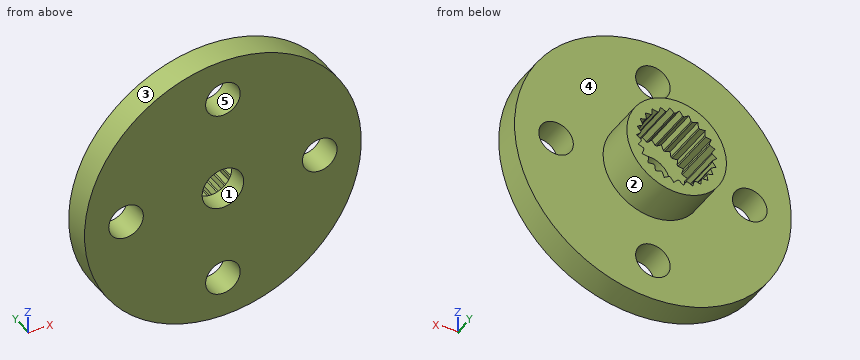
```python
from build123d import *

# Parameters (mm, degrees)
M3_TAPPED_HOLE1_D  = 2.5
CUT_EXTRUDE1_DEPTH = 3.5


with BuildPart() as part:
    # Sketch1 → Revolve1 (revolve)
    with BuildSketch(Plane.XY, mode=Mode.PRIVATE) as revolve1_sk:
        Polygon((2.345142076, 2), (1.5, 2), (1.5, 0), (10, 0), (10, 2), (3.6, 2), (3.6, 5), (2.345142076, 5), align=None)
    revolve(revolve1_sk.sketch.rotate(Axis((0, 6.795271061, 0), (0, -1, 0)), 90), axis=Axis((0, 6.795271061, 0), (0, -1, 0)))

    # M3 Tapped Hole1 (through all)
    with Locations(Plane(origin=(0, 2, 0), x_dir=(1, 0, 0), z_dir=(0, 1, 0))):
        with Locations((-7, 0), (0, 7), (7, 0), (0, -7)):
            Hole(M3_TAPPED_HOLE1_D / 2)

    # Sketch5 → Cut-Extrude1 (cut)
    with BuildSketch(Plane(origin=(0, 5, 0), x_dir=(1, 0, 0), z_dir=(0, 1, 0))):
        Polygon((-1.365561553, 2.212519298), (-1.76486465, 2.301141622), (-1.782802347, 1.892515731), (-1.855371341, 1.821427239), (-2.264280127, 1.811914873), (-2.18390601, 1.410870135), (-2.237353692, 1.324480448), (-2.632103873, 1.217386217), (-2.458088994, 0.847229896), (-2.489309178, 0.750559669), (-2.846959309, 0.552107499), (-2.589416781, 0.234351734), (-2.596595063, 0.133019089), (-2.896359819, -0.1452577), (-2.570257076, -0.392146098), (-2.552976281, -0.492252076), (-2.777434424, -0.834181049), (-2.401723373, -0.995853825), (-2.360987798, -1.08891534), (-2.497094635, -1.474624828), (-2.093610237, -1.541686147), (-2.031787285, -1.622294803), (-2.071632783, -2.029368772), (-1.663824084, -1.997921274), (-1.584506681, -2.061392388), (-1.525775164, -2.466173179), (-1.137342523, -2.338044479), (-1.045140308, -2.380689341), (-0.891245038, -2.759652566), (-0.544762749, -2.542289037), (-0.445034179, -2.561629282), (-0.20491899, -2.892750976), (0.079476656, -2.598784997), (0.180935719, -2.593696641), (0.493316205, -2.857733214), (0.699097167, -2.504249019), (0.79639029, -2.475027779), (1.162881655, -2.656634385), (1.278088691, -2.264175191), (1.365561553, -2.212519298), (1.76486465, -2.301141622), (1.782802347, -1.892515731), (1.855371341, -1.821427239), (2.264280127, -1.811914873), (2.18390601, -1.410870135), (2.237353692, -1.324480448), (2.632103873, -1.217386217), (2.458088994, -0.847229896), (2.489309178, -0.750559669), (2.846959309, -0.552107499), (2.589416781, -0.234351734), (2.596595063, -0.133019089), (2.896359819, 0.1452577), (2.570257076, 0.392146098), (2.552976281, 0.492252076), (2.777434424, 0.834181049), (2.401723373, 0.995853825), (2.360987798, 1.08891534), (2.497094635, 1.474624828), (2.093610237, 1.541686147), (2.031787285, 1.622294803), (2.071632783, 2.029368772), (1.663824084, 1.997921274), (1.584506681, 2.061392388), (1.525775164, 2.466173179), (1.137342523, 2.338044479), (1.045140308, 2.380689341), (0.891245038, 2.759652566), (0.544762749, 2.542289037), (0.445034179, 2.561629282), (0.20491899, 2.892750976), (-0.079476656, 2.598784997), (-0.180935719, 2.593696641), (-0.493316205, 2.857733214), (-0.699097167, 2.504249019), (-0.79639029, 2.475027779), (-1.162881655, 2.656634385), (-1.278088691, 2.264175191), align=None)
    extrude(amount=-CUT_EXTRUDE1_DEPTH, mode=Mode.SUBTRACT)


solid = part.part
```
Geometry check sheet. Reference: the model listing, model coordinates, mm. Face numbers are marked on the shaded views. A direction names the side the tool comes from. Give positions to 0.01 mm unless a question says otherwise; leave off trailing zeros. Loops run counter-clockwise (first coordinate to the right, second up) from the corner with the lowest first, then second, coordinate; pieces in that order, holes last. Notation, with made-up numbers: (25.25, 54.25) - (66.25, 54.25) arc R28 ccw to (66.25, 84.25) - close; hole circle Ø6 at (-15, 79.5). An arc over 180 degrees is marked (long way). Use CSV: the item, a comma, the result in double quotes. Start each with the question number.
Q1. Section check D-D, the plane z = -8.5. Record the cut outline in (x, y).
Q2. Section check B-B, the plane z = 8. Record the cut outline in (x, y).
Q3. Scan lines: probe 1 along Y at (x, z) = (6, 1); probe 2 along Z at (x, y) = (-6.25, 0.35); probe 3 along Y at (x, z) = (1, -1.25). Record each from-to range of solid material in increasing order. Write a range as from..to.
Q4. Section check A-A, the plane x = 8. Record the cut outline in (y, z), and give its area (3 significant figures).
Q5. Section check C-C, the plane y = 0.45. Record the cut outline in (x, z), and give its area (3 significant figures).
Q6. Release check for a two-part mould opening along X. For the marked faces 3, 4 and 5 record: +X half, -X half, draft (parallel to the pull), parting line (faces both ways), or undercut.
Q7. Access from +Z, -Z, +X, -X, +Y, -Y to the whole of each face (thin tool, end or side, straight path). Record for the marked faces 1 and 2.
Q8. Go/stop test with flat-tipped pins: pin 1 Ø3 at (x, z) = (-7, 0) entering from +Y; pin 2 Ø2 at (x, y) = (-5.5, 2) entering from +Z; pin 3 Ø3 at (y, z) = (1.5, -6.5) entering from -X; pin 4 Ø1.5 at (x, z) = (7, 0) entering from -Y. Record where each tip stops, or that it passes through.
Findings below:
1,outline,"(-5.27, 0) - (5.27, 0) - (5.27, 2) - (-5.27, 2) - close"
2,outline,"(-6, 0) - (-0.75, 0) - (-0.75, 2) - (-6, 2) - close; (0.75, 0) - (6, 0) - (6, 2) - (0.75, 2) - close"
3,probe 1,"y = 0..2"
3,probe 2,"z = -7.81..-1, 1..7.81"
3,probe 3,"y = 0..1.5"
4,outline,"(0, -6) - (2, -6) - (2, -0.75) - (0, -0.75) - close; (0, 0.75) - (2, 0.75) - (2, 6) - (0, 6) - close"
4,area,"21.0 mm^2"
5,outline,"circle Ø20 at (0, 0); hole circle Ø2.5 at (-7, 0); hole circle Ø3 at (0, 0); hole circle Ø2.5 at (0, -7); hole circle Ø2.5 at (0, 7); hole circle Ø2.5 at (7, 0)"
5,area,"287 mm^2"
6,face 3,"parting line"
6,face 4,"draft"
6,face 5,"undercut"
7,face 1,"+Y, -Y"
7,face 2,"+Y"
8,pin 1,"stops at y = 2"
8,pin 2,"stops at z = 8.93"
8,pin 3,"stops at x = -8.66"
8,pin 4,"passes through"
